The drawing under review shows one solid part. Ordinate dimensions are in mm from its lowest x, y, z. Coordinates: 2 decimals unless noted, no trailing zeros. Order: outer loops, then holes, each group sorted by start corner. A loop starts at its lowest first (then second) coordinate and runs counter-clockwise, first axis right, second up. Notation, with made-up numbers: (-5.75, 6) - (16.25, 6) arc R15 cw to (16.25, 12) - close; hole circle Ø10 at (-4.75, 61). An arc over 180 degrees is marked (long way). Write each question's results on one line, items separated by ' | '. Start each with the question number.
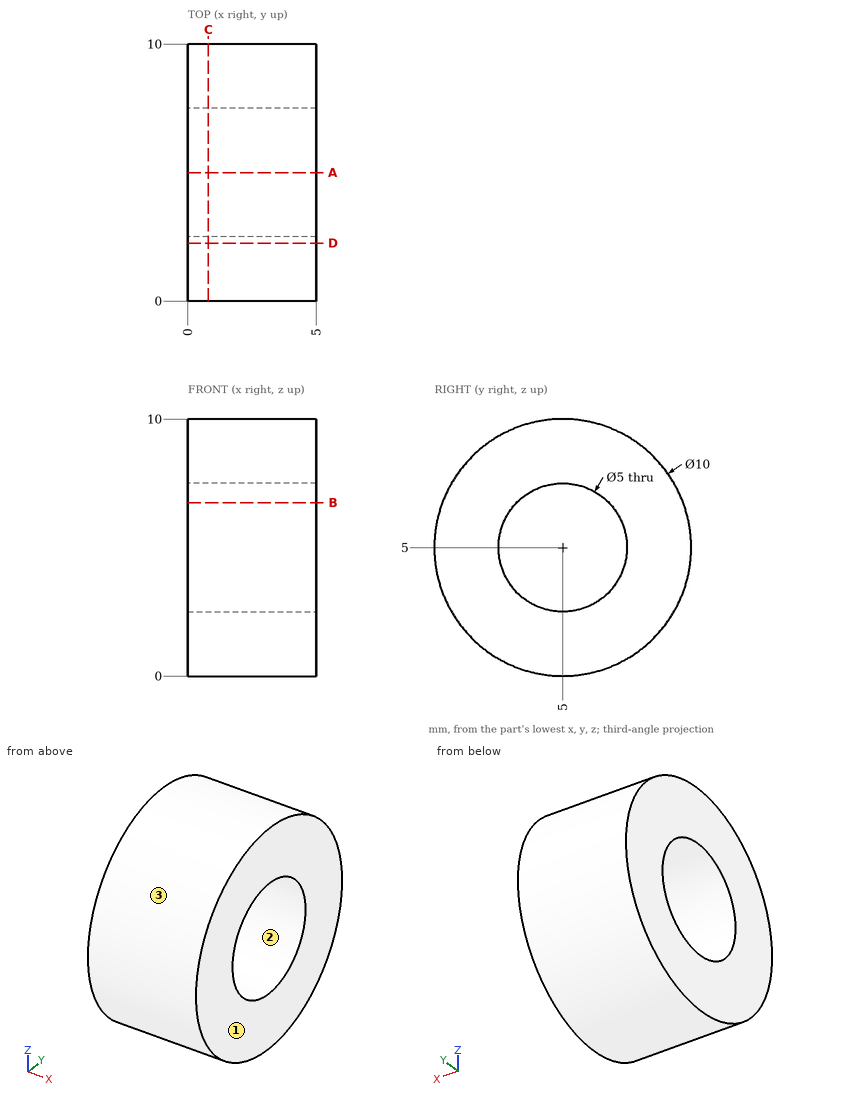
(1) To check wall thickness, follow line 1 along Y through (x, z) = (2.75, 5); line 2 along Z through (x, y) = (2.9, 4.5); line 3 along Y through (x, z) = (3.45, 2.75). State the ranges of each line that lie inside material, in increasing order. Write a range as [from, to].
(2) Take a section at A-A (y = 5). State the section outline as (x, z) points.
(3) Mouldability with a two-part tool opening along Y and no side actions: class the marked faces 1, 2 and 3 as +Y half, -Y half, draft (parallel to the pull), parting line (faces both ways), or undercut.
(4) Take a section at C-C (x = 0.8). State the section outline as (y, z) points, plus the area to 3 significant figures.
(5) Clearance check with a flat-ended pin moving along its axis: pin 1 (3 mm diameter, centred on x = 4, z = 1.5, fed in from -Y). State where the tip first meets the part, or that it passes through.
(6) Take a section at B-B (z = 6.75). State the section outline as (x, y) points, plus the area to 3 significant figures.
(7) Take a section at D-D (y = 2.25). State the section outline as (x, z) points.
Worked out:
1) line 1: [0, 2.5], [7.5, 10] | line 2: [0.03, 2.55], [7.45, 9.97] | line 3: [0.53, 3.91], [6.09, 9.47]
2) outline: (0, 0) - (5, 0) - (5, 2.5) - (0, 2.5) - close; (0, 7.5) - (5, 7.5) - (5, 10) - (0, 10) - close
3) face 1: draft | face 2: undercut | face 3: parting line
4) outline: circle Ø10 at (5, 5); hole circle Ø5 at (5, 5) | area: 58.9 mm^2
5) pin 1: y = 0.42
6) outline: (0, 0.32) - (5, 0.32) - (5, 3.21) - (0, 3.21) - close; (0, 6.79) - (5, 6.79) - (5, 9.68) - (0, 9.68) - close | area: 29.0 mm^2
7) outline: (0, 0.82) - (5, 0.82) - (5, 9.18) - (0, 9.18) - close
